from build123d import *

# Parameters (mm, degrees)
SKETCH1_W               = 100
SKETCH1_H               = 100
SKETCH1_W_2             = 96
SKETCH1_H_2             = 96
EXTRUDE_THIN1_DEPTH     = 29
SKETCH2_W               = 100
SKETCH2_H               = 100
BOSS_EXTRUDE1_DEPTH     = 2
CUT_EXTRUDE1_REACH      = 92.2
CUT_EXTRUDE2_DEPTH      = 160
CUT_EXTRUDE3_DEPTH      = 160
CHAMFER1_SIZE           = 1
CUT_EXTRUDE4_DEPTH      = 116.503246708
CUT_EXTRUDE4_DEPTH_BACK = 116.503246708
SKETCH7_R               = 4.15
SKETCH8_R               = 2.5
CUT_EXTRUDE5_DEPTH      = 177


with BuildPart() as part:
    # Sketch1 → Extrude-Thin1 (new, symmetric)
    with BuildSketch(Plane.XY):
        Rectangle(SKETCH1_W, SKETCH1_H)
        Rectangle(SKETCH1_W_2, SKETCH1_H_2, mode=Mode.SUBTRACT)
    extrude(amount=EXTRUDE_THIN1_DEPTH, both=True)

    # Sketch2 → Boss-Extrude1 (add)
    with BuildSketch(Plane(origin=(0, 0, -29), x_dir=(-1, 0, 0), z_dir=(0, 0, -1))):
        Rectangle(SKETCH2_W, SKETCH2_H)
    extrude(amount=-BOSS_EXTRUDE1_DEPTH)

    # Sketch3 → Cut-Extrude1 (cut, up to next)
    with BuildSketch(Plane.XY.offset(-27), mode=Mode.PRIVATE) as cut_extrude1_sk1:
        with BuildLine():
            Line((-20.5, -23), (-20.5, 10))
            Line((-20.5, 10), (20.5, 10))
            Line((20.5, 10), (20.5, -23))
            ThreePointArc((20.5, -23), (0, -43.5), (-20.5, -23))
        make_face()
    cut_extrude1_tool1 = extrude(cut_extrude1_sk1.sketch, amount=-CUT_EXTRUDE1_REACH, mode=Mode.PRIVATE) & part.part
    add(cut_extrude1_tool1.solids().sort_by_distance((0, -14.763519, -27))[0], mode=Mode.SUBTRACT)

    # Sketch4 → Cut-Extrude2 (cut)
    with BuildSketch(Plane.ZY.offset(50)):
        with BuildLine():
            Line((11.6, 1), (11.6, -13))
            ThreePointArc((11.6, -13), (9, -15.6), (6.4, -13))
            Line((6.4, -13), (6.4, 1))
            ThreePointArc((6.4, 1), (9, 3.6), (11.6, 1))
        make_face()
    extrude(amount=-CUT_EXTRUDE2_DEPTH, mode=Mode.SUBTRACT)

    # Sketch6 → Cut-Extrude3 (cut)
    with BuildSketch(Plane(origin=(0, 0, -29), x_dir=(-1, 0, 0), z_dir=(0, 0, -1))):
        with BuildLine():
            Line((-2.6, 10), (-2.6, 30))
            ThreePointArc((-2.6, 30), (0, 32.6), (2.6, 30))
            Line((2.6, 30), (2.6, 10))
            ThreePointArc((2.6, 10), (0, 7.4), (-2.6, 10))
        make_face()
    extrude(amount=-CUT_EXTRUDE3_DEPTH, mode=Mode.SUBTRACT)

    # Chamfer1
    chamfer1_edges = [part.edges().sort_by_distance(p)[0] for p in [
        (-2.6, 10, -28),
        (2.6, 10, -28),
    ]]
    chamfer(chamfer1_edges, length=CHAMFER1_SIZE)

    # Sketch7 → Cut-Extrude4 (cut, two sides: drawn at the far end of the back side and taken through both)
    with BuildSketch(Plane(origin=(0, 50, 0), x_dir=(1, 0, 0), z_dir=(0, 1, 0)).offset(-CUT_EXTRUDE4_DEPTH_BACK)):
        with Locations(Location((-34, 1, 0), (0, 0, 270))):
            Circle(SKETCH7_R)
        with Locations(Location((34, 1, 0), (0, 0, 270))):
            Circle(SKETCH7_R)
    extrude(amount=CUT_EXTRUDE4_DEPTH + CUT_EXTRUDE4_DEPTH_BACK, mode=Mode.SUBTRACT)

    # Sketch8 → Cut-Extrude5 (cut)
    with BuildSketch(Plane(origin=(0, 50, 0), x_dir=(1, 0, 0), z_dir=(0, 1, 0))):
        with Locations(Location((-34, 17, 0), (0, 0, 270))):
            Circle(SKETCH8_R)
        with Locations(Location((-34, -15, 0), (0, 0, 270))):
            Circle(SKETCH8_R)
        with Locations(Location((34, 17, 0), (0, 0, 270))):
            Circle(SKETCH8_R)
        with Locations(Location((34, -15, 0), (0, 0, 270))):
            Circle(SKETCH8_R)
    extrude(amount=-CUT_EXTRUDE5_DEPTH, mode=Mode.SUBTRACT)


solid = part.part
Design review of the part built by this model. Coordinates are the model's own, in mm. A direction names the side the tool comes from. Round coordinates to 2 decimals unless told otherwise and drop trailing zeros. Write each loop counter-clockwise with the first axis right and the second up, starting at its lowest first coordinate (ties: lowest second). Pieces come first, ordered by that corner, then holes. Notation, with made-up numbers: (-32, 19.5) -> (25, 19.5) arc R16 cw to (25, 24.5) -> close; hole circle Ø4 at (28.5, 45.5). An arc over 180 degrees is marked (long way). One line per item, written item: value. Start each with the question number.
Q1. Tool access review of faces 1 (the face through (0.451, -43.495, -27.986)), 2 (the face through (-1, -48, 1)), 3 (the face through (49, 3.6, 8.9)): name each direction out of +Z, -Z, +X, -X, +Y, -Y from which nothing blocks a thin tool from reaching the whole face with its end or side.
Q2. Add section D-D (z = 9). Give the boundary of the cut face in (x, y).
Q3. Add section B-B (z = 15). Give the boundary of the cut face in (x, y), then the cut area to 3 significant figures.
Q4. To check wall thickness, follow probe 1 along X at (y, z) = (-49.05, -1); probe 2 along X at (y, z) = (48.9, -17); probe 3 along Y at (x, z) = (-1.5, -6). State the ranges of each line that lie inside material, in increasing order.
Q5. Insertion check: P1, Ø10, axis at x = 23.5, y = 30, coming from the +Z side. The pin has a flat end and moves straight along its axis. Give the tip position at first contact, or say it passes through.
Q6. Add section A-A (y = 26.5). Give the boundary of the cut face in (x, z), then the cut area to 3 significant figures.
Q7. Add section C-C (x = -24). Give the boundary of the cut face in (y, z).
Q8. The part is to be moulded in two halves that separate along X. For faces 4 (the face through (-48, -1, 1)), 5 (the face through (-49, -15.6, 9.1)), 6 (the face through (48, -1, 1)), say which applies: pulls with the +X half, pulls with the -X half, needs draft (parallel to the pull), parting line crosses it, or undercut.
Response:
1. face 1: +Z, -Z
1. face 2: +Z
1. face 3: +X, -X
2. outline: (-50, -50) -> (50, -50) -> (50, -15.6) -> (48, -15.6) -> (48, -48) -> (-48, -48) -> (-48, -15.6) -> (-50, -15.6) -> close; (-50, 3.6) -> (-48, 3.6) -> (-48, 48) -> (48, 48) -> (48, 3.6) -> (50, 3.6) -> (50, 50) -> (-50, 50) -> close
3. outline: (-50, -50) -> (-36.5, -50) -> (-36.5, -48) -> (-48, -48) -> (-48, 48) -> (-36.5, 48) -> (-36.5, 50) -> (-50, 50) -> close; (-31.5, -50) -> (31.5, -50) -> (31.5, -48) -> (-31.5, -48) -> close; (-31.5, 48) -> (31.5, 48) -> (31.5, 50) -> (-31.5, 50) -> close; (36.5, -50) -> (50, -50) -> (50, 50) -> (36.5, 50) -> (36.5, 48) -> (48, 48) -> (48, -48) -> (36.5, -48) -> close
3. area: 744 mm^2
4. probe 1: x = -50 to -38.15, -29.85 to 29.85, 38.15 to 50
4. probe 2: x = -50 to -36.5, -31.5 to 31.5, 36.5 to 50
4. probe 3: y = -50 to -48, 48 to 50
5. P1: stops at z = -27
6. outline: (-50, -29) -> (-2.6, -29) -> (-2.6, -27) -> (-48, -27) -> (-48, 29) -> (-50, 29) -> close; (2.6, -29) -> (50, -29) -> (50, 29) -> (48, 29) -> (48, -27) -> (2.6, -27) -> close
6. area: 414 mm^2
7. outline: (-50, -29) -> (50, -29) -> (50, 29) -> (48, 29) -> (48, -27) -> (-48, -27) -> (-48, 29) -> (-50, 29) -> close
8. face 4: undercut
8. face 5: needs draft
8. face 6: undercut
